Here's how the part is built. I have some questions about the finished solid (model axes, mm). A direction names the side the tool comes from. Coordinates: 2 decimals unless noted, no trailing zeros. Order: outer loops, then holes, each group sorted by start corner. A loop starts at its lowest first (then second) coordinate and runs counter-clockwise, first axis right, second up. Notation, with made-up numbers: (66, 76.5) -> (74, 76.5) arc R19 cw to (74, 89.5) -> close; hole circle Ø2 at (-9.75, 64). An arc over 180 degrees is marked (long way). One line per item, written item: value. Start each with the question number.
```python
from build123d import *

# Parameters (mm, degrees)
SKETCH1_R               = 7.62
BOSS_EXTRUDE1_DEPTH     = 1.27
BOSS_EXTRUDE2_DEPTH     = 7.62
SKETCH4_R               = 6.35
BOSS_EXTRUDE3_DEPTH     = 2.54
SKETCH5_R               = 2
CUT_EXTRUDE1_DEPTH      = 1
CUT_EXTRUDE1_DEPTH_BACK = 12.43


with BuildPart() as part:
    # Sketch1 → Boss-Extrude1 (new body)
    with BuildSketch(Plane.XY):
        Circle(SKETCH1_R)
    extrude(amount=BOSS_EXTRUDE1_DEPTH)

    # Sketch2 → Boss-Extrude2 (add)
    with BuildSketch(Plane.XY.offset(1.27)):
        Polygon((4.917620463, -5.438781327), (7.168933026, 1.539393583), (2.251312563, 6.97817491), (-4.917620463, 5.438781327), (-7.168933026, -1.539393583), (-2.251312563, -6.97817491), align=None)
    extrude(amount=BOSS_EXTRUDE2_DEPTH)

    # Sketch4 → Boss-Extrude3 (add)
    with BuildSketch(Plane.XY.offset(8.89)):
        Circle(SKETCH4_R)
    extrude(amount=BOSS_EXTRUDE3_DEPTH)

    # Sketch5 → Cut-Extrude1 (cut, two sides)
    with BuildSketch(Plane.XY.offset(11.43)) as cut_extrude1_sk:
        Circle(SKETCH5_R)
    extrude(amount=CUT_EXTRUDE1_DEPTH, mode=Mode.SUBTRACT)
    extrude(cut_extrude1_sk.sketch, amount=-CUT_EXTRUDE1_DEPTH_BACK, mode=Mode.SUBTRACT)


solid = part.part
```
Q1. Imagine slicing it at A-A (z = 5.25). Write out the boundary of the cut face in (x, y), plus the area to 3 significant figures.
Q2. Imagine slicing it at B-B (x = 0). Write out the boundary of the cut face in (y, z), plus the area to 3 significant figures.
Q3. For faces 1 (the face through (-6.028, 1.999, 5.027)), 2 (the face through (-4.745, -4.221, 5.027)), 3 (the face through (2.2, -6.2, 1.27)), 4 (the face through (4.4, -4.9, 8.89)), which set-ups out of +Z, -Z, +X, -X, +Y, -Y let a thin tool reach every point of the face, with its end or its side?
Q4. Imagine slicing it at C-C (y = 0). Write out the boundary of the cut face in (x, z).
Q5. I need wall thicknesses on line 1 (Y direction, x = 0, z = 9); line 2 (Y direction, x = 0, z = 6.75); line 3 (Z direction, x = -0.75, y = 6.5). Which ranges of each line are inside material? Lowest first, please.
Q6. For P1, Ø6, axis at y = 6, z = 7, coming from the -X side; P2, Ø1.5, axis at y = 0.5, z = 9.5, coming from the -X side; P3, Ø4, axis at y = 5, z = 8.5, coming from the +X side, each with a flat end and sliding along its axis, tell me the tip position at first contact or that it passes through.
Completed:
1. outline: (-7.17, -1.54) -> (-2.25, -6.98) -> (4.92, -5.44) -> (7.17, 1.54) -> (2.25, 6.98) -> (-4.92, 5.44) -> close; hole circle Ø4 at (0, 0)
1. area: 127 mm2
2. outline: (-7.62, 0) -> (-2, 0) -> (-2, 11.43) -> (-6.35, 11.43) -> (-6.35, 8.89) -> (-6.49, 8.89) -> (-6.49, 1.27) -> (-7.62, 1.27) -> close; (2, 0) -> (7.62, 0) -> (7.62, 1.27) -> (6.49, 1.27) -> (6.49, 8.89) -> (6.35, 8.89) -> (6.35, 11.43) -> (2, 11.43) -> close
2. area: 105 mm2
3. face 1: +Z, -X, +Y
3. face 2: +Z, -X, -Y
3. face 3: +Z
3. face 4: +Z, +X, -Y
4. outline: (-7.62, 0) -> (-2, 0) -> (-2, 11.43) -> (-6.35, 11.43) -> (-6.35, 8.89) -> (-6.67, 8.89) -> (-6.67, 1.27) -> (-7.62, 1.27) -> close; (2, 0) -> (7.62, 0) -> (7.62, 1.27) -> (6.67, 1.27) -> (6.67, 8.89) -> (6.35, 8.89) -> (6.35, 11.43) -> (2, 11.43) -> close
5. line 1: y = -6.35 to -2, 2 to 6.35
5. line 2: y = -6.49 to -2, 2 to 6.49
5. line 3: z = 0 to 1.27
6. P1: stops at x = -5.7
6. P2: stops at x = -6.65
6. P3: stops at x = 5.85
